Model file for the job. Use its own axes, mm. A direction names the side the tool comes from. Round coordinates to 2 decimals unless told otherwise and drop trailing zeros. Loops run counter-clockwise (first coordinate to the right, second up) from the corner with the lowest first, then second, coordinate; pieces in that order, holes last. Notation, with made-up numbers: (15.25, 42) -> (45.25, 42) arc R6 cw to (45.25, 48) -> close; hole circle Ø9 at (79, 52.5). An arc over 180 degrees is marked (long way). Use a Markdown table: item, result.
from build123d import *

# Parameters (mm, degrees)
F1_W     = 8
F1_H     = 30
F1_R     = 2.2
F2_DEPTH = 5
F0_W     = 30
F0_H     = 8
F0_R     = 2.2
F3_DEPTH = 5
F5_SIZE  = 15
F4_R     = 2.1
F6_DEPTH = 30


with BuildPart() as f2:
    # F1 (on Right) → F2 (new body)
    with BuildSketch(Plane.YZ):
        with Locations((20, 15)):
            Rectangle(F1_W, F1_H)
        with Locations((12, 15)):
            Rectangle(F1_W, F1_H)
        with Locations((12.000000596, 25)):
            Circle(F1_R, mode=Mode.SUBTRACT)
        with Locations((4, 15)):
            Rectangle(F1_W, F1_H)
    extrude(amount=F2_DEPTH)

    # F0 (on Top) → F3 (join)
    with BuildSketch(Plane.XY):
        with Locations((15, 20)):
            Rectangle(F0_W, F0_H)
        with Locations((15, 12)):
            Rectangle(F0_W, F0_H)
        with Locations((25, 12)):
            Circle(F0_R, mode=Mode.SUBTRACT)
        with Locations((15, 4)):
            Rectangle(F0_W, F0_H)
    extrude(amount=F3_DEPTH)

    # F5
    f5_edges = [f2.edges().sort_by_distance(p)[0] for p in [
        (5, 12, 5),
    ]]
    chamfer(f5_edges, length=F5_SIZE)

    # F4 (on Front) → F6 (cut)
    with BuildSketch(Plane.XZ):
        with BuildLine():
            Line((8.9047972998, 2.3616264964), (17.6383735036, 2.3616264964))
            Line((17.6383735036, 2.3616264964), (11.929701132, 8.070298868))
            ThreePointArc((11.929701132, 8.070298868), (12.0160710439, 7.5396825646), (12.0449723862, 7.0028603077))
            ThreePointArc((12.0449723862, 7.0028603077), (11.1861753858, 4.2009970498), (8.9047972998, 2.3616264964))
        make_face()
        with BuildLine():
            ThreePointArc((2.6568189153, 9.3995474202), (4.970273692, 11.5521047865), (8.1124109465, 11.8875890535))
            Line((8.1124109465, 11.8875890535), (2.6568189153, 17.3431810847))
            Line((2.6568189153, 17.3431810847), (2.6568189153, 9.3995474202))
        make_face()
        with Locations((7.0449723862, 7.0028603077)):
            Circle(F4_R)
    extrude(amount=-F6_DEPTH, mode=Mode.SUBTRACT)


solid = f2.part
Q1. Flat gauge pins, fed straight in: pin 1 (1 mm diameter, centred on x = 21, y = 7.5, fed in from +Z); pin 2 (3 mm diameter, centred on x = 16, y = 14, fed in from +Z); pin 3 (8 mm diameter, centred on y = 8, z = 25.5, fed in from +X). Where does each tip first touch, or does it go through?
Results list:
| item | result |
|---|---|
| pin 1 | stops at z = 5 |
| pin 2 | stops at z = 10.5 |
| pin 3 | stops at x = 5 |
Q2. Band-saw the part on C-C, the plane y = 6. Give the cut face in (x, z).
Results list:
| item | result |
|---|---|
| outline | (0, 0) -> (30, 0) -> (30, 5) -> (20, 5) -> (5, 20) -> (5, 30) -> (0, 30) -> close; hole (2.66, 9.4) arc R5 cw to (8.11, 11.89) -> (2.66, 17.34) -> close; hole circle Ø4.2 at (7.04, 7); hole (8.9, 2.36) -> (17.64, 2.36) -> (11.93, 8.07) arc R5 cw to start |
Q3. Band-saw the part on B-B, the plane x = 25. Give the cut face in (y, z).
Results list:
| item | result |
|---|---|
| outline | (0, 0) -> (9.8, 0) -> (9.8, 5) -> (0, 5) -> close; (14.2, 0) -> (24, 0) -> (24, 5) -> (14.2, 5) -> close |
Q4. Drill centre lines: L1, parallel to Y at x = 25, z = 3.6; L2, parallel to Z at x = 6, y = 9.75; L3, parallel to X at y = 9.5, z = 29. Where is each one in solid material? Low to high. Write a range as from..to.
Results list:
| item | result |
|---|---|
| L1 | y = 0..9.8, 14.2..24 |
| L2 | z = 0..5.18, 8.82..11.89, 14..19 |
| L3 | x = 0..5 |
Q5. Band-saw the part on A-A, the plane y = 12. Give the cut face in (x, z).
Results list:
| item | result |
|---|---|
| outline | (0, 0) -> (22.8, 0) -> (22.8, 5) -> (20, 5) -> (5, 20) -> (5, 22.8) -> (0, 22.8) -> close; (0, 27.2) -> (5, 27.2) -> (5, 30) -> (0, 30) -> close; (27.2, 0) -> (30, 0) -> (30, 5) -> (27.2, 5) -> close; hole (2.66, 9.4) arc R5 cw to (8.11, 11.89) -> (2.66, 17.34) -> close; hole circle Ø4.2 at (7.04, 7); hole (8.9, 2.36) -> (17.64, 2.36) -> (11.93, 8.07) arc R5 cw to start |
Q6. Tool access for faces 1 (the face through (25, 15, 5)), 2 (the face through (11, 0, 11)), 3 (the face through (13, 12, 2.362)): list every direction of +Z, -Z, +X, -X, +Y, -Y with a clear straight run to the whole face (end or side of a thin tool).
Results list:
| item | result |
|---|---|
| face 1 | +Z, +X, +Y, -Y |
| face 2 | +Z, -Z, +X, -X, -Y |
| face 3 | +Y, -Y |
Q7. Pull direction Z, two halves, no side cores. Call faces 4 (the face through (15, 12, 0)), 5 (the face through (11, 24, 11)), 6 (the face through (4.929, 11.832, 11.533)): released by +Z, released by -Z, zero draft, split by the parting line, or undercut.
Results list:
| item | result |
|---|---|
| face 4 | released by -Z |
| face 5 | zero draft |
| face 6 | undercut |
Q8. Band-saw the part on D-D, the plane z = 25. Give the cut face in (x, y), plus the area to 3 significant figures.
Results list:
| item | result |
|---|---|
| outline | (0, 0) -> (5, 0) -> (5, 9.8) -> (0, 9.8) -> close; (0, 14.2) -> (5, 14.2) -> (5, 24) -> (0, 24) -> close |
| area | 98.0 mm² |
